Here's how the part is built. I have some questions about the finished solid (model axes, mm). A direction names the side the tool comes from. Give positions to 0.01 mm unless a question says otherwise; leave off trailing zeros. Loops run counter-clockwise (first coordinate to the right, second up) from the corner with the lowest first, then second, coordinate; pieces in that order, holes last. Notation, with made-up numbers: (-36.5, 60) -> (19.5, 60) arc R3 ccw to (19.5, 65) -> close; hole circle Ø11 at (-33, -12.75). An arc over 180 degrees is marked (long way). Answer in a Markdown table with one row per item. Add a question column.
Item 1: Which directions (+Z, -Z, +X, -X, +Y, -Y) give clear straight access to the entire face, cutting with the end or side of a thin tool? Please do faces 4 (the face through (123.825, 38, 26)), 5 (the face through (143, 25, 12.54)), 6 (the face through (-37.846, 25, -120)), 7 (the face through (0, 23, -55)), 8 (the face through (-7.62, 48, -49)).
Item 2: If we section it at D-D (z = -120.65): Write out the boundary of the cut face in (x, y).
Item 3: If we section it at A-A (z = 25.4): Write out the boundary of the cut face in (x, y) (3 decimals), then the cut area to 3 significant figures.
Item 4: If I drill on line 1 (X direction, y = 49.45, z = 25.4) (3 decimals); line 2 (X direction, y = 43.5, z = 25.4) (3 decimals); line 3 (Z direction, x = 116.5, y = 42), over which ranges is the centre line in solid material (lowest first)?
Item 5: If we section it at C-C (y = 29.5): Write out the boundary of the cut face in (x, z) (3 decimals), then the cut area to 3 significant figures.
Item 6: We'd pull the mould along Y, two halves only. Please class faces 1 (the face through (114.3, 38.2, 44.5)), 2 (the face through (149.21, 48.41, 28.7)), 3 (the face through (31, 0, 6)): released by +Y, released by -Y, zero draft, split by the parting line, or undercut.
Item 7: For P1, Ø7.5, axis at x = -22, z = -118, coming from the -Y side; P2, Ø10, axis at y = 13.5, z = -7, coming from the +X side; P3, Ø3, axis at x = 122, y = 45, coming from the -Z side, each with a flat end and sliding along its axis, tell me the tip position at first contact or that it passes through.
Item 8: If we section it at B-B (x = -25.4): Write out the boundary of the cut face in (y, z), then the cut area to 3 significant figures.
```python
from build123d import *

# Parameters (mm, degrees)
BOSS_EXTRUDE1_DEPTH = 50.8
SKETCH3_W           = 25.4
SKETCH3_H           = 25.4
CUT_EXTRUDE1_DEPTH  = 25.4
SKETCH8_W           = 24.892
SKETCH8_H           = 24.892
BOSS_EXTRUDE2_DEPTH = 24.892
SKETCH12_R          = 3.429
CUT_EXTRUDE2_DEPTH  = 25.4
SKETCH13_W          = 12.7
SKETCH13_H          = 25.4
CUT_EXTRUDE3_DEPTH  = 25.908
FILLET1_R           = 2.54
CUT_EXTRUDE6_DEPTH  = 5.08
SKETCH15_R          = 3.175
CUT_EXTRUDE7_DEPTH  = 246.984968624


with BuildPart() as part:
    # Sketch2 → Boss-Extrude1 (new body)
    with BuildSketch(Plane(origin=(0, 0, 0), x_dir=(1, 0, 0), z_dir=(0, 1, 0))):
        Polygon((-50.8, 107.95), (0, 107.95), (0, 0), (155.575, 0), (155.575, -50.8), (-50.8, -50.8), align=None)
    extrude(amount=BOSS_EXTRUDE1_DEPTH)

    # Sketch3 → Cut-Extrude1 (cut)
    with BuildSketch(Plane(origin=(155.575, 0, 0), x_dir=(0, 0, -1), z_dir=(1, 0, 0))):
        with Locations((-25.239912, 25.560088)):
            Rectangle(SKETCH3_W, SKETCH3_H)
    extrude(amount=-CUT_EXTRUDE1_DEPTH, mode=Mode.SUBTRACT)

    # Sketch7 → CBORE for 1/4 Binding Head Machine Screw1 (revolve, cut)
    with BuildSketch(Plane(origin=(142.875, 50.8, 25.4), x_dir=(0, 0, 1), z_dir=(1, 0, 0))):
        Polygon((0, 0), (0, 50.8), (3.3782, 50.8), (3.3782, 4.191), (7.14375, 4.191), (7.14375, 0.635), (7.77875, 0), align=None)
    revolve(axis=Axis((142.875, 57.15, 25.4), (0, -1, 0)), mode=Mode.SUBTRACT)

    # Sketch8 → Boss-Extrude2 (add)
    with BuildSketch(Plane(origin=(0, 0, -107.95), x_dir=(-1, 0, 0), z_dir=(0, 0, -1))):
        with Locations((25.4, 25.4)):
            Rectangle(SKETCH8_W, SKETCH8_H)
    extrude(amount=BOSS_EXTRUDE2_DEPTH)

    # Sketch12 → Cut-Extrude2 (cut)
    with BuildSketch(Plane(origin=(0, 37.846, 0), x_dir=(1, 0, 0), z_dir=(0, 1, 0))):
        with Locations(Location((-25.4, 120.65, 0), (0, 0, 270))):
            Circle(SKETCH12_R)
    extrude(amount=-CUT_EXTRUDE2_DEPTH, mode=Mode.SUBTRACT)

    # Sketch13 → Cut-Extrude3 (cut)
    with BuildSketch(Plane(origin=(0, 50.8, 0), x_dir=(1, 0, 0), z_dir=(0, 1, 0))):
        with Locations((117.475, -25.4)):
            Rectangle(SKETCH13_W, SKETCH13_H)
    extrude(amount=-CUT_EXTRUDE3_DEPTH, mode=Mode.SUBTRACT)

    # Fillet1
    fillet1_edges = [part.edges().sort_by_distance(p)[0] for p in [
        (117.475, 50.8, 12.7),
        (117.475, 50.8, 38.1),
    ]]
    fillet(fillet1_edges, radius=FILLET1_R)

    # Sketch17 → Cut-Extrude6 (cut)
    with BuildSketch(Plane(origin=(0, 50.8, 0), x_dir=(1, 0, 0), z_dir=(0, 1, 0))):
        Polygon((0, 107.95), (0, 0), (155.575, 0), (155.575, -7.62), (-7.62, -7.62), (-7.62, 107.95), align=None)
    extrude(amount=-CUT_EXTRUDE6_DEPTH, mode=Mode.SUBTRACT)

    # Sketch15 → Cut-Extrude7 (cut, through all)
    with BuildSketch(Plane.XY.offset(50.8)):
        with Locations((117.475, 38.1)):
            Circle(SKETCH15_R)
    extrude(amount=-CUT_EXTRUDE7_DEPTH, mode=Mode.SUBTRACT)


solid = part.part
```
Recorded:
| question | item | result |
|---|---|---|
| 1 | face 4 | +Y |
| 1 | face 5 | +X |
| 1 | face 6 | -Z, -X, +Y, -Y |
| 1 | face 7 | -Z, +X, +Y, -Y |
| 1 | face 8 | -Z, +X, +Y |
| 2 | outline | (-37.85, 12.95) -> (-28.83, 12.95) -> (-28.83, 37.85) -> (-37.85, 37.85) -> close; (-21.97, 12.95) -> (-12.95, 12.95) -> (-12.95, 37.85) -> (-21.97, 37.85) -> close |
| 3 | outline | (-50.8, 0) -> (139.497, 0) -> (139.497, 12.86) -> (130.175, 12.86) -> (130.175, 38.26) -> (139.497, 38.26) -> (139.497, 46.609) -> (135.731, 46.609) -> (135.731, 50.165) -> (135.096, 50.8) -> (123.825, 50.8) -> (123.825, 24.892) -> (111.125, 24.892) -> (111.125, 50.8) -> (-50.8, 50.8) -> close; (146.253, 0) -> (155.575, 0) -> (155.575, 12.86) -> (146.253, 12.86) -> close; (146.253, 38.26) -> (155.575, 38.26) -> (155.575, 50.8) -> (150.654, 50.8) -> (150.019, 50.165) -> (150.019, 46.609) -> (146.253, 46.609) -> close |
| 3 | area | 9,310 mm^2 |
| 4 | line 1 | x = -50.8 to 111.125, 123.825 to 135.731, 150.019 to 155.575 |
| 4 | line 2 | x = -50.8 to 111.125, 123.825 to 139.497, 146.253 to 155.575 |
| 4 | line 3 | z = 0 to 12.7, 38.1 to 50.8 |
| 5 | outline | (-50.8, -107.95) -> (-37.846, -107.95) -> (-37.846, -132.842) -> (-12.954, -132.842) -> (-12.954, -107.95) -> (0, -107.95) -> (0, 0) -> (155.575, 0) -> (155.575, 12.54) -> (130.175, 12.54) -> (130.175, 37.94) -> (155.575, 37.94) -> (155.575, 50.8) -> (-50.8, 50.8) -> close; hole circle Ø6.858 at (-25.4, -120.65); hole (111.125, 12.7) -> (123.825, 12.7) -> (123.825, 38.1) -> (111.125, 38.1) -> close |
| 5 | area | 15,600 mm^2 |
| 6 | face 1 | undercut |
| 6 | face 2 | zero draft |
| 6 | face 3 | released by -Y |
| 7 | P1 | stops at y = 12.95 |
| 7 | P2 | stops at x = 0 |
| 7 | P3 | stops at z = 0 |
| 8 | outline | (0, -107.95) -> (12.95, -107.95) -> (12.95, -117.22) -> (37.85, -117.22) -> (37.85, -107.95) -> (50.8, -107.95) -> (50.8, 50.8) -> (0, 50.8) -> close; (12.95, -132.84) -> (37.85, -132.84) -> (37.85, -124.08) -> (12.95, -124.08) -> close |
| 8 | area | 8,510 mm^2 |
